Autodesk Fusion 360 part; units mm, degrees
sketch "Schizzo1" plane through (0, 0, 0) normal (1, 0, 0) x (0, 1, 0)
  line L0 (20.1, -10.1) -> (-20.1, -10.1)
  line L1 (-20.1, -10.1) -> (-20.1, 10.1)
  line L2 (-20.1, 10.1) -> (20.1, 10.1)
  line L3 (20.1, 10.1) -> (20.1, -10.1)
  line L4 (20.1, -10.1) -> (-20.1, 10.1) construction
  line L5 (-20.1, -10.1) -> (20.1, 10.1) construction
  line L6 (-60, -40) -> (60, -40)
  line L7 (60, -40) -> (60, 40)
  line L8 (60, 40) -> (-60, 40)
  line L9 (-60, 40) -> (-60, -40)
  line L10 (-60, -40) -> (60, 40) construction
  line L11 (60, -40) -> (-60, 40) construction
  dimension "d1" = 40.2
  dimension "d2" = 20.2
  dimension "d3" = 120
  dimension "d4" = 80
extrude "Estrusione1" add sketch "Schizzo1" along normal blind 10
sketch "Schizzo2" plane through (10, 0, 0) normal (1, 0, 0) x (0, 1, 0)
  line L0 (-20.1, 10.1) -> (20.1, 10.1)
  line L1 (20.1, 10.1) -> (20.1, -10.1)
  line L2 (20.1, -10.1) -> (-20.1, -10.1)
  line L3 (-20.1, -10.1) -> (-20.1, 10.1)
  line L4 (-60, 40) -> (-60, -40)
  line L5 (-60, -40) -> (60, -40)
  line L6 (60, -40) -> (60, 40)
  line L7 (60, 40) -> (-60, 40)
  line L8 (-20.1, -10.1) -> (20.1, -10.1)
  line L9 (20.1, -10.1) -> (20.1, 10.1)
  line L10 (20.1, 10.1) -> (-20.1, 10.1)
  line L11 (-20.1, 10.1) -> (-20.1, -10.1)
  line L12 (-20.1, -10.1) -> (20.1, 10.1) construction
  line L13 (20.1, -10.1) -> (-20.1, 10.1) construction
  line L14 (-30, -20) -> (30, -20)
  line L15 (30, -20) -> (30, 20)
  line L16 (30, 20) -> (-30, 20)
  line L17 (-30, 20) -> (-30, -20)
  line L18 (-30, -20) -> (30, 20) construction
  line L19 (30, -20) -> (-30, 20) construction
  dimension "d7" = 60
  dimension "d8" = 40
extrude "Estrusione2" add sketch "Schizzo2" along normal blind 50 contours L14 L15 L16 L17
sketch "Schizzo3" plane through (0, 0, -20) normal (0, 0, -1) x (1, 0, 0)
  line L0 (10, 30) -> (10, -30)
  line L1 (10, -30) -> (60, -30)
  line L2 (60, -30) -> (60, 30)
  line L3 (60, 30) -> (10, 30)
  line L4 (60, 0) -> (0, 0) construction
  line L5 (60, -10) -> (0, -10) construction
  circle A0 centre (50, -10) radius 2.5
  circle A1 centre (25, -10) radius 2.5
  circle A2 centre (50, 10) radius 2.5
  circle A3 centre (25, 10) radius 2.5
  point P0 (35, -10)
  dimension "d11" = 10
  dimension "d12" = 5
  dimension "d13" = 5
  dimension "d14" = 25
  dimension "d15" = 15
  dimension "d16" = 25
extrude "Estrusione3" cut sketch "Schizzo3" against normal blind 43 contours A0 | A1 | A2 | A3
sketch "Schizzo4" plane through (10, 0, 0) normal (1, 0, 0) x (0, 1, 0)
  line L0 (-30, 20) -> (30, 20)
  line L1 (30, 20) -> (30, -20)
  line L2 (30, -20) -> (-30, -20)
  line L3 (-30, -20) -> (-30, 20)
  line L4 (-60, 40) -> (-60, -40)
  line L5 (-60, -40) -> (60, -40)
  line L6 (60, -40) -> (60, 40)
  line L7 (60, 40) -> (-60, 40)
  line L8 (0, 40) -> (0, -40) construction
  line L9 (45, -40) -> (45, 40)
  circle A0 centre (45, 0) radius 2.5
  circle A1 centre (45, -25) radius 2.5
  circle A2 centre (45, 25) radius 2.5
  circle A3 centre (-45, -25) radius 2.5
  circle A4 centre (-45, 0) radius 2.5
  circle A5 centre (-45, 25) radius 2.5
  dimension "d19" = 5
  dimension "d20" = 5
  dimension "d21" = 5
  dimension "d22" = 25
  dimension "d23" = 25
extrude "Estrusione4" cut sketch "Schizzo4" against normal blind 25 contours L9 A2 | L9 A2 | L9 A1 | L9 A1 | L9 A0 | L9 A0 | A3 | A4 | A5
fillet "Raccordo1" radius 5 4 edges at (5, 60, -40) (5, 60, 40) (5, -60, 40) (5, -60, -40)
fillet "Raccordo2" radius 6 4 edges at (10, 0, 20) (10, -30, 0) (10, 30, 0) (10, 0, -20)
fillet "Raccordo3" radius 1.5 8 edges at (60, 20.1, 0) (60, 0, -10.1) (60, 0, 10.1) (60, -20.1, 0) (60, -30, 0) (60, 0, 20) (60, 30, 0) (60, 0, -20)
Design review of the part built by this model. Coordinates are the model's own, in mm. A direction names the side the tool comes from. Coordinates: 2 decimals unless noted, no trailing zeros. Loops run counter-clockwise (first coordinate to the right, second up) from the corner with the lowest first, then second, coordinate; pieces in that order, holes last. Notation, with made-up numbers: (67.25, -0.75) -> (110.25, -0.75) arc R21 ccw to (110.25, 11.25) -> close; hole circle Ø7 at (-33.75, 14). An arc over 180 degrees is marked (long way). Answer as a JSON object with one key per item and string values.
Q1. Take a section at B-B on y = 10. Give the number of separate pieces and of enclosed holes in the cut face, plus the area to 3 significant figures.
Answer block:
{"separate pieces": "6", "enclosed holes": "0", "area": "1,400 mm^2"}
Q2. To check wall thickness, follow L1, parallel to Y at x = 25, z = 13; L2, parallel to X at y = -10, z = -12; L3, parallel to Z at x = 2.5, y = 45. State the ranges of each line that lie inside material, in increasing order.
Answer block:
{"L1": "y = -30 to -12.5, -7.5 to 7.5, 12.5 to 30", "L2": "x = 0 to 22.5, 27.5 to 47.5, 52.5 to 60", "L3": "z = -40 to -27.5, -22.5 to -2.5, 2.5 to 22.5, 27.5 to 40"}
Q3. Clearance check with flat-ended pins moving along their axes: pin 1 Ø4 at (y, z) = (-6, -29.5) entering from +X; pin 2 Ø3 at (x, y) = (27, 14) entering from -Z; pin 3 Ø6 at (x, y) = (51.5, -3.5) entering from +Z; pin 4 Ø3 at (x, y) = (50, -10) entering from -Z. State where each tip first meets the part, or that it passes through.
Answer block:
{"pin 1": "stops at x = 10", "pin 2": "stops at z = -20", "pin 3": "stops at z = 20", "pin 4": "passes through"}
Q4. Take a section at C-C on x = 54.5. Give the boundary of the cut face in (y, z), plus the area to 3 significant figures.
Answer block:
{"outline": "(-30, -20) -> (30, -20) -> (30, 20) -> (-30, 20) -> close; hole (-20.1, -10.1) -> (20.1, -10.1) -> (20.1, 10.1) -> (-20.1, 10.1) -> close", "area": "1,590 mm^2"}
Q5. The part is to be moulded in two halves that separate along Y. For faces 5 (the cylindrical face through (52.31, 10.96, 14.98)), 6 (the cylindrical face through (5, -58, 39)), 7 (the cylindrical face through (11.711, 31.804, 0.364)), 8 (the cylindrical face through (5.07, -43.66, -22.89)), say which applies: +Y half, -Y half, draft (parallel to the pull), parting line (faces both ways), or undercut.
Answer block:
{"face 5": "undercut", "face 6": "-Y half", "face 7": "+Y half", "face 8": "undercut"}
Q6. Take a section at D-D on z = -16.5. Give the boundary of the cut face in (x, y).
Answer block:
{"outline": "(0, -60) -> (10, -60) -> (10, -36) arc R6 cw to (16, -30) -> (58.5, -30) arc R1.5 ccw to (60, -28.5) -> (60, 28.5) arc R1.5 ccw to (58.5, 30) -> (16, 30) arc R6 cw to (10, 36) -> (10, 60) -> (0, 60) -> close; hole circle Ø5 at (25, -10); hole circle Ø5 at (25, 10); hole circle Ø5 at (50, -10); hole circle Ø5 at (50, 10)"}
Q7. Take a section at A-A on z = 0. Give the boundary of the cut face in (x, y), plus the area to 3 significant figures.
Answer block:
{"outline": "(0, -60) -> (10, -60) -> (10, -47.5) -> (0, -47.5) -> close; (0, -42.5) -> (10, -42.5) -> (10, -36) arc R6 cw to (16, -30) -> (58.5, -30) arc R1.5 ccw to (60, -28.5) -> (60, -21.6) arc R1.5 ccw to (58.5, -20.1) -> (0, -20.1) -> close; (0, 20.1) -> (58.5, 20.1) arc R1.5 ccw to (60, 21.6) -> (60, 28.5) arc R1.5 ccw to (58.5, 30) -> (16, 30) arc R6 cw to (10, 36) -> (10, 42.5) -> (0, 42.5) -> close; (0, 47.5) -> (10, 47.5) -> (10, 60) -> (0, 60) -> close", "area": "1,700 mm^2"}
Q8. Tool access review of faces 1 (the flat face through (37, -30, 0)), 2 (the flat face through (29, 20.1, 0)), 3 (the flat face through (10, -1, 27)), 4 (the flat face through (37, 30, 0)): name each direction out of +Z, -Z, +X, -X, +Y, -Y from which nothing blocks a thin tool from reaching the whole face with its end or side.
Answer block:
{"face 1": "+Z, -Z, +X, -Y", "face 2": "+X, -X", "face 3": "+X", "face 4": "+Z, -Z, +X, +Y"}
